Geometry check sheet. Reference: the model listing, model coordinates, mm. A direction names the side the tool comes from. Coordinates: 2 decimals unless noted, no trailing zeros. Loops run counter-clockwise (first coordinate to the right, second up) from the corner with the lowest first, then second, coordinate; pieces in that order, holes last. Notation, with made-up numbers: (7, -39.75) - (28, -39.75) arc R18 ccw to (28, -7.75) - close; hole circle Ø10 at (0, 31). An arc over 180 degrees is marked (long way). One line per item, written item: value.
Autodesk Inventor part; units mm, degrees
ref_plane "YZ Plane" through (0, 0, 0) normal (1, 0, 0) x (0, 1, 0)
ref_plane "XZ Plane" through (0, 0, 0) normal (0, 1, 0) x (-1, 0, 0)
ref_plane "XY Plane" through (0, 0, 0) normal (0, 0, 1) x (1, 0, 0)
sketch "Sketch1" plane through (0, 0, 0) normal (0, 0, 1) x (1, 0, 0)
  line L0 (0, 0) -> (150, 0)
  line L1 (150, 0) -> (150, 100)
  line L2 (150, 100) -> (0, 100)
  line L3 (0, 100) -> (0, 0)
  dimension "d0" = 150
  dimension "d1" = 100
extrude "Extrusion1" add sketch "Sketch1" along normal blind 250
fillet "Fillet1" radius 20 1 edges at (150, 100, 125)
fillet "Fillet2" radius 20 1 edges at (150, 0, 125)
fillet "Fillet3" radius 20 1 edges at (0, 100, 125)
fillet "Fillet4" radius 20 1 edges at (0, 0, 125)
fillet "Fillet5" radius 5 8 edges at (5.8579, 94.1421, 0) (0, 50, 0) (5.8579, 5.8579, 0) (75, 0, 0) (144.1421, 5.8579, 0) (150, 50, 0) (144.1421, 94.1421, 0) (75, 100, 0)
sketch "Sketch2" plane through (20, 0, 250) normal (0, -1, 0) x (1, 0, 0)
  line L0 (110, 0) -> (110, -245)
  line L1 (0, -245) -> (0, 0)
  line L2 (110, -171.6757) -> (0, -171.6757)
  line L3 (0, -171.6757) -> (0, -166.6757)
  line L4 (0, -166.6757) -> (110, -166.6757)
  line L5 (110, -166.6757) -> (110, -171.6757)
  line L6 (95.3863, -226.2308) -> (70.3863, -226.2308)
  line L7 (70.3863, -226.2308) -> (70.3863, -221.2308)
  line L8 (70.3863, -221.2308) -> (95.3863, -221.2308)
  line L9 (95.3863, -221.2308) -> (95.3863, -226.2308)
  line L10 (37.9599, -226.2308) -> (12.9599, -226.2308)
  line L11 (12.9599, -226.2308) -> (12.9599, -221.2308)
  line L12 (12.9599, -221.2308) -> (37.9599, -221.2308)
  line L13 (37.9599, -221.2308) -> (37.9599, -226.2308)
  line L14 (27.9599, -236.2308) -> (22.9599, -236.2308)
  line L15 (22.9599, -236.2308) -> (22.9599, -211.2308)
  line L16 (22.9599, -211.2308) -> (27.9599, -211.2308)
  line L17 (27.9599, -211.2308) -> (27.9599, -236.2308)
  point P0 (-20, -250)
  point P1 (27.9599, -226.2308)
  point P2 (27.9599, -221.2308)
  point P3 (22.9599, -221.2308)
  point P4 (22.9599, -226.2308)
  dimension "d9" = 25
  dimension "d10" = 5
  dimension "d11" = 5
  dimension "d12" = 25
  dimension "d13" = 10
  dimension "d14" = 10
  dimension "d15" = 5
  dimension "d16" = 25
  dimension "d17" = 5
extrude "Extrusion2" add sketch "Sketch2" along normal blind 5
sketch "Sketch3" plane through (0, 0, 0) normal (0, 0, -1) x (-1, 0, 0)
  line L0 (-20, 100) -> (-130, 100)
  line L1 (-150, 80) -> (-150, 20)
  circle A0 centre (-110, 50) radius 12.5
  circle A1 centre (-40, 51.4507) radius 12.5
  point P0 (0, 0)
  point P1 (-150, 50)
  dimension "d20" = 50
  dimension "d21" = 40
  dimension "d22" = 70
  dimension "d23" = 25
  dimension "d24" = 25
extrude "Extrusion3" add sketch "Sketch3" along normal blind 3
sketch "Sketch4" plane through (110, 50, -3) normal (0, 0, -1) x (-1, 0, 0)
  circle A0 centre (0, 0) radius 7.2404
  circle A1 centre (70, 1.4507) radius 12.5
  circle A2 centre (70, 1.4507) radius 7.5
  point P0 (110, -50)
  dimension "d27" = 15
extrude "Extrusion4" add sketch "Sketch4" along normal blind 15 contours A0 | A2
sketch "Sketch5" plane through (110, 50, -18) normal (0, 0, -1) x (-1, 0, 0)
  circle A0 centre (0, 0) radius 7.2404
  circle A1 centre (0, 0) radius 10
  circle A2 centre (70, 1.4507) radius 7.5
  circle A3 centre (70, 1.4507) radius 8.5
  point P0 (110, -50)
  dimension "d30" = 20
  dimension "d31" = 17
extrude "Extrusion5" add sketch "Sketch5" along normal blind 4 contours A0 | A1 | A2 | A3
sketch "Sketch6" plane through (110, 50, -22) normal (0, 0, -1) x (-1, 0, 0)
  circle A0 centre (0, 0) radius 10
  point P0 (110, -50)
hole "Hole1" at (110, 50, -22) direction (0, 0, 1) diameter 10.106 depth 28 tip angle 118
sketch "Sketch7" plane through (40, 51.4507, -22) normal (0, 0, -1) x (-1, 0, 0)
  circle A0 centre (0, 0) radius 8.5
  point P0 (40, -51.4507)
hole "Hole2" at (40, 51.4507, -22) direction (0, 0, 1) diameter 10.647 depth 28 tip angle 118
sketch "Sketch8" plane through (0, 20, 250) normal (-1, 0, 0) x (0, 0, 1)
  line L0 (-245, 80) -> (-245, 60)
  line L1 (-245, 60) -> (-73.5714, 60) construction
  line L2 (-73.5714, 60) -> (-73.5714, 0) construction
  line L3 (-73.5714, 0) -> (-245, 0) construction
  line L4 (-245, 0) -> (-245, 60) construction
  line L5 (-245, 0) -> (-245, 60)
  point P0 (-250, -20)
decal "Decal1"
sketch "Sketch9" plane through (20, 100, 250) normal (0, 1, 0) x (1, 0, 0)
  line L0 (0, 250) -> (110, 250)
  circle A0 centre (57.15, 250) radius 9.5
  point P0 (-20, 250)
  dimension "d50" = 19
sketch "Sketch10" plane through (20, 0, 5) normal (0, -1, 0) x (1, 0, 0)
  line L0 (0, -5) -> (110, -5)
  circle A0 centre (57.15, -5) radius 9.5
  point P0 (-20, -5)
  point P1 (66.65, -5)
  point P2 (47.65, -5)
  dimension "d51" = 19
extrude "Extrusion6" cut sketch "Sketch10" against normal blind 50 contours A0 L0 picked at (56.7683, -1.8564)
properties part number "battery eg 26"
(1) Cross-section at B-B on x = 77.15. Record the cut outline in (y, z).
Reply:
outline: (-5, 78.32) - (0, 78.32) - (0, 9.5) - (50, 9.5) - (50, 0) - (95, 0) arc R5 ccw to (100, 5) - (100, 250) - (0, 250) - (0, 83.32) - (-5, 83.32) - close
(2) Cross-section at A-A on z = 106.5. Record the cut outline in (x, y), and give its area (3 significant figures).
Reply:
outline: (0, 20) arc R20 ccw to (20, 0) - (130, 0) arc R20 ccw to (150, 20) - (150, 80) arc R20 ccw to (130, 100) - (20, 100) arc R20 ccw to (0, 80) - close
area: 14,700 mm2
(3) Cross-section at C-C on y = 33. Record the cut outline in (x, z), and give its area (3 significant figures).
Reply:
outline: (0, 5) arc R5 ccw to (5, 0) - (67.65, 0) arc R9.5 cw to (86.65, 0) - (145, 0) arc R5 ccw to (150, 5) - (150, 250) - (0, 250) - close
area: 37,300 mm2
(4) Release check for a two-part mould opening along X. For faces 6 (the face through (53, -2, 28.769)), 7 (the face through (57.96, -2, 26)), 8 (the face through (144.297, 93.986, 129.215)) record: pulls with the +X half, pulls with the -X half, needs draft (parallel to the pull), parting line crosses it, or undercut.
Reply:
face 6: needs draft
face 7: undercut
face 8: pulls with the +X half
(5) Access from +Z, -Z, +X, -X, +Y, -Y to the whole of each face (thin tool, end or side, straight path). Record for faces 1 (the face through (77.359, 24.65, 9.498)), 2 (the face through (74, 51, 0)), 3 (the face through (40, 43, -3)), 4 (the face through (74, 0, 165)), 5 (the face through (115.386, -2, 26)).
Reply:
face 1: -Z, -Y
face 2: -Z
face 3: none
face 4: +Z, +X, -X, -Y
face 5: -Z, +X, -Y
(6) Go/stop test with flat-tipped pins: pin 1 Ø1 at (x, y) = (69, 59) entering from -Z; pin 2 Ø6 at (x, y) = (110, 50) entering from -Z; pin 3 Ø1 at (y, z) = (8.5, 34) entering from -X. Record where each tip stops, or that it passes through.
Reply:
pin 1: z = 0
pin 2: z = 7.23
pin 3: x = 3.3
(7) Material ranges on probe 1 along Z at (x, y) = (116, 45.5); probe 2 along Y at (x, z) = (40, -2); probe 3 along Y at (x, z) = (95, 178), recorded low to high. Write a range as from..to.
Reply:
probe 1: -22..-18, -3..250
probe 2: 38.95..46.13, 56.77..63.95
probe 3: 0..100
